Drawing for the job (mm, zero at the part's lowest x, y, z). Round coordinates to 2 decimals unless told otherwise and drop trailing zeros. Write each loop counter-clockwise with the first axis right and the second up, starting at its lowest first coordinate (ties: lowest second). Pieces come first, ordered by that corner, then holes. Notation, with made-up numbers: (-15, -23.5) -> (15, -23.5) arc R17 cw to (15, 2.5) -> close; hole circle Ø6 at (85, -4.5). An arc over 180 degrees is marked (long way). One line per question, with ' | ' between items.
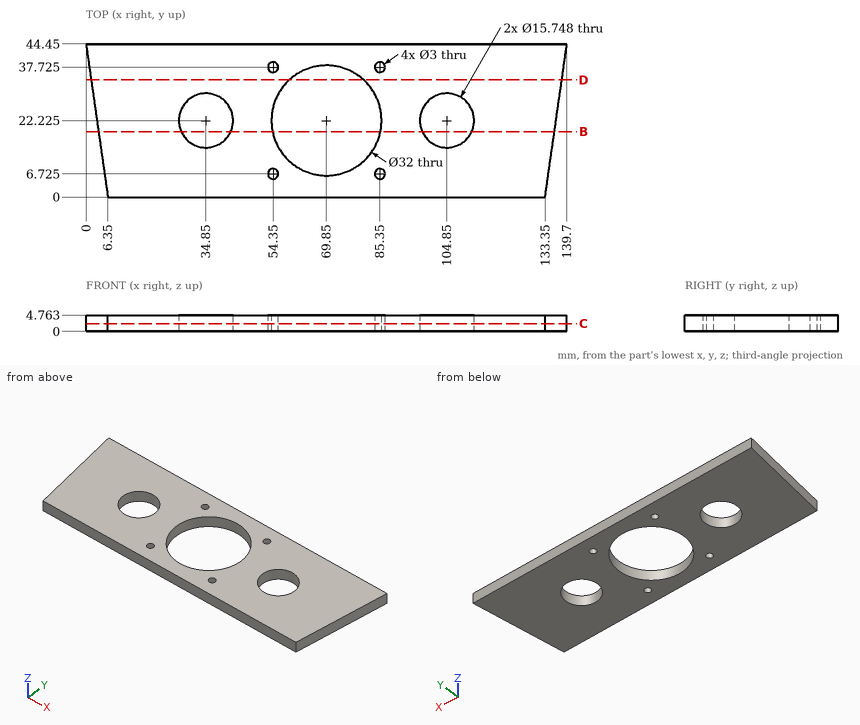
(1) Wall check: line 1 (Y direction, x = 34.85, z = 2.25); line 2 (X direction, y = 8, z = 4.45) (1 decimal); line 3 (X direction, y = 5.5, z = 1.25) (1 decimal). Give the ranges that are in metal, low to high. Write a range as from..to.
Calculated:
line 1: 0..14.35, 30.1..44.45 | line 2: 5.2..53.6, 55.1..62.5, 77.2..84.6, 86.1..134.5 | line 3: 5.6..53.5, 55.2..84.5, 86.2..134.1
(2) Slice it at D-D (y = 34). Write the cut outline in (x, z), then the cut area to 3 significant figures.
Calculated:
outline: (1.49, 0) -> (59.02, 0) -> (59.02, 4.76) -> (1.49, 4.76) -> close; (80.68, 0) -> (138.21, 0) -> (138.21, 4.76) -> (80.68, 4.76) -> close | area: 548 mm2
(3) Drop flat-ended pins along their axis: pin 1 (1.5 mm diameter, centred on y = 10.5, z = 3.5, fed in from +X); pin 2 (1 mm diameter, centred on y = 10, z = 4, fed in from -X). Give the stop position or say it passes through.
Calculated:
pin 1: x = 134.96 | pin 2: x = 4.85
(4) Slice it at B-B (y = 19). Write the cut outline in (x, z) (1 decimal).
Calculated:
outline: (3.6, 0) -> (27.7, 0) -> (27.7, 4.8) -> (3.6, 4.8) -> close; (42, 0) -> (54.2, 0) -> (54.2, 4.8) -> (42, 4.8) -> close; (85.5, 0) -> (97.7, 0) -> (97.7, 4.8) -> (85.5, 4.8) -> close; (112, 0) -> (136.1, 0) -> (136.1, 4.8) -> (112, 4.8) -> close
(5) Slice it at C-C (z = 2.3). State how many separate pieces and enclosed holes the cut face has.
Calculated:
separate pieces: 1 | enclosed holes: 7
